Verification items for the finished model (mm, model axes). A direction names the side the tool comes from. Round coordinates to 2 decimals unless told otherwise and drop trailing zeros. Write each loop counter-clockwise with the first axis right and the second up, starting at its lowest first coordinate (ties: lowest second). Pieces come first, ordered by that corner, then holes. Notation, with made-up numbers: M -33.75,42.25 L -14.75,42.25 A14 ccw -14.75,52.25 Z; hole C 14,78 d7. An arc over 180 degrees is marked long. Answer in a Markdown table with one row per item. Add a question column.
1. Set-up check for faces 1 (the flat face through (-19, 1, 0)), 2 (the flat face through (-44, -8, 6.096)): record each of +Z, -Z, +X, -X, +Y, -Y from which the full face is reachable in a straight line by a thin tool's end or side.
2. Go/stop test with flat-tipped pins: pin 1 Ø2 at (x, z) = (-21.5, 1.5) entering from -Y; pin 2 Ø0.6 at (y, z) = (16, 6.5) entering from -X; pin 3 Ø0.6 at (y, z) = (30, 6.5) entering from -X. Record where each tip stops, or that it passes through.
3. Material ranges on probe 1 along Y at (x, z) = (-38, 6.25); probe 2 along Z at (x, y) = (13.5, -2); probe 3 along Z at (x, y) = (4, -14.5), recorded low to high.
4. Sectioned sample at A-A on y = 19. Record the cut outline in (x, z), plus the area to 3 significant figures.
5. Draft check along X on faces 3 (the flat face through (-55.315, 1.596, 3.219)), 4 (the flat face through (0, 21, 6.604)), 5 (the flat face through (-23, 13, 6.096)), 6 (the flat face through (-44, 28, 6.096)). Enter one of: pulls with the +X half, pulls with the -X half, needs draft (parallel to the pull), parting line crosses it, or undercut.
```python
from build123d import *

# Parameters (mm, degrees)
F0_W     = 38.1
F0_H     = 76.2
F1_DEPTH = 6.35
F3_DEPTH = 6.35
F5_W     = 8.6051712304
F5_H     = 10.1246496194
F6_DEPTH = 0.254
F8_DEPTH = 0.254


with BuildPart() as f1:
    # F0 (on Top) → F1 (new body)
    with BuildSketch(Plane.XY):
        Rectangle(F0_W, F0_H)
    extrude(amount=F1_DEPTH)

    # F2 (on face) → F3 (cut)
    with BuildSketch(Plane.XY.offset(6.35)):
        with BuildLine():
            Line((-3.9472845383, 38.1), (-3.8636967831, 38.1))
            add(Edge.make_bspline(
                [(-3.9472845383, 38.1), (-3.9204592136, 38.1251084892), (-3.8998782769, 38.127174182), (-3.8636967831, 38.1)],
                knots=[0.4563634252, 0.4563634252, 0.4563634252, 0.4563634252, 0.4871979804, 0.4871979804, 0.4871979804, 0.4871979804], degree=3))
        make_face()
        with BuildLine():
            add(Edge.make_bspline(
                [(-19.05, 32.5106605887), (-6.1091777888, 32.3092094071), (-4.3443097915, 37.7283845811), (-3.9472845383, 38.1)],
                knots=[0, 0, 0, 0, 0.4563634252, 0.4563634252, 0.4563634252, 0.4563634252], degree=3))
            Line((-3.9472845383, 38.1), (-19.05, 38.1))
            Line((-19.05, 38.1), (-19.05, 32.5106605887))
        make_face()
        with BuildLine():
            Line((19.05, -38.1), (19.05, 3.1485415529))
            Line((19.05, 3.1485415529), (15.3276119381, 0))
            add(Edge.make_bspline(
                [(15.3276119381, 0), (15.1655543596, -11.4850010723), (13.7070389464, -32.0684760809), (-13.3565291762, -32.3926247656)],
                knots=[0, 0, 0, 0, 43.2673328352, 43.2673328352, 43.2673328352, 43.2673328352], degree=3))
            Line((-13.3565291762, -32.3926247656), (-19.05, -38.1))
            Line((-19.05, -38.1), (19.05, -38.1))
        make_face()
        with BuildLine():
            Line((19.05, 3.1485415529), (19.05, 32.5106605887))
            ThreePointArc((19.05, 32.5106605887), (12.2820636744, 17.8296010708), (19.05, 3.1485415529))
        make_face()
        Polygon((15.2206547403, 38.1), (19.05, 32.5106605887), (19.05, 38.1), align=None)
        with BuildLine():
            add(Edge.make_bspline(
                [(-3.8636967831, 38.1), (-3.843737622, 38.0850096328), (-3.0988894532, 37.3648301618), (5.2937592339, 27.6119129043), (15.2206547403, 38.1)],
                knots=[0.4871979804, 0.4871979804, 0.4871979804, 0.4871979804, 0.5042075561, 1, 1, 1, 1], degree=3))
            Line((15.2206547403, 38.1), (-3.8636967831, 38.1))
        make_face()
    extrude(amount=-F3_DEPTH, mode=Mode.SUBTRACT)

    # F4: F1 across face


with BuildPart() as f1_1:
    add(f1.part)
    add(f1.part.mirror(Plane(origin=(-19.05, -2.7946697056, 3.175), x_dir=(0, -1, 0), z_dir=(-1, 0, 0))))

    # F5 (on face) → F6 (cut)
    with BuildSketch(Plane.XY.offset(6.35)):
        with BuildLine():
            ThreePointArc((-37.5772565603, 32.5917619335), (-45.671204203, 31.008244813), (-53.4049263852, 33.873389857))
            ThreePointArc((-53.4049263852, 33.873389857), (-50.1581802259, 29.7090041206), (-47.9535559256, 24.9107647687))
            Line((-47.9535559256, 24.9107647687), (-37.5772565603, 24.9107647687))
            Line((-37.5772565603, 24.9107647687), (-37.5772565603, 32.5917619335))
        make_face()
        with BuildLine():
            Line((-37.5772565603, 17.7330877632), (-46.8293691707, 17.7330877632))
            ThreePointArc((-46.8293691707, 17.7330877632), (-47.4515529833, 12.5316587806), (-49.2414900542, 7.6084381438))
            Line((-49.2414900542, 7.6084381438), (-37.5772565603, 7.6084381438))
            Line((-37.5772565603, 7.6084381438), (-37.5772565603, 17.7330877632))
        make_face()
        with Locations((-23.3525856152, 12.6707629535)):
            Rectangle(F5_W, F5_H)
        with BuildLine():
            add(Edge.make_bspline(
                [(-27.6551712304, 30.7719508767), (-25.0542603527, 29.9722405749), (-22.0663375313, 29.5693060648), (-19.05, 29.5798139295)],
                knots=[8.2498540023, 8.2498540023, 8.2498540023, 8.2498540023, 15.7954011192, 15.7954011192, 15.7954011192, 15.7954011192], degree=3))
            Line((-27.6551712304, 30.7719508767), (-27.6551712304, 24.9107647687))
            Line((-27.6551712304, 24.9107647687), (-19.05, 24.9107647687))
            Line((-19.05, 24.9107647687), (-19.05, 29.5798139295))
        make_face()
        with BuildLine():
            add(Edge.make_bspline(
                [(-14.7775728256, 29.8755089086), (-13.3218013512, 30.0752082684), (-11.9002315961, 30.3766424012), (-10.555408895, 30.7817886934)],
                knots=[19.3738855113, 19.3738855113, 19.3738855113, 19.3738855113, 23.0815953476, 23.0815953476, 23.0815953476, 23.0815953476], degree=3))
            Line((-14.7775728256, 29.8755089086), (-14.7775728256, 7.6084381438))
            Line((-14.7775728256, 7.6084381438), (-10.555408895, 7.6084381438))
            Line((-10.555408895, 7.6084381438), (-10.555408895, 30.7817886934))
        make_face()
        with BuildLine():
            add(Edge.make_bspline(
                [(-6.3332454301, 32.5660842134), (-5.2855915186, 33.1701122102), (-4.348215472, 33.8675739108), (-3.5563470113, 34.6601066929)],
                knots=[27.291897076, 27.291897076, 27.291897076, 27.291897076, 30.7735982336, 30.7735982336, 30.7735982336, 30.7735982336], degree=3))
            Line((-6.3332454301, 32.5660842134), (-6.3332454301, 7.6084381438))
            Line((-6.3332454301, 7.6084381438), (-2.1110819653, 7.6084381438))
            Line((-2.1110819653, 7.6084381438), (-2.1110819653, 33.5563536252))
            ThreePointArc((-2.1110819653, 33.5563536252), (-2.8501925125, 34.0866536733), (-3.5563470113, 34.6601066929))
        make_face()
        with BuildLine():
            ThreePointArc((6.3332458958, 30.9586713834), (4.2005089038, 31.1180342806), (2.1110812668, 31.5743847599))
            Line((2.1110812668, 31.5743847599), (2.1110812668, 7.6084381438))
            Line((2.1110812668, 7.6084381438), (6.3332458958, 7.6084381438))
            Line((6.3332458958, 7.6084381438), (6.3332458958, 30.9586713834))
        make_face()
        with BuildLine():
            Line((11.1414900542, 0), (2.5332975201, 0))
            Line((2.5332975201, 0), (2.5332975201, -21.0394149611))
            add(Edge.make_bspline(
                [(2.5332975201, -21.0394149611), (7.0844292813, -16.8218684935), (10.3040141885, -10.1988507211), (11.1414900542, 0)],
                knots=[0.7794890643, 0.7794890643, 0.7794890643, 0.7794890643, 1, 1, 1, 1], degree=3))
        make_face()
        with BuildLine():
            Line((-6.1221369542, 0), (-14.7775728256, 0))
            Line((-14.7775728256, 0), (-14.7775728256, -6.1859292111))
            ThreePointArc((-14.7775728256, -6.1859292111), (-12.0094062526, -9.1081265301), (-11.0027304346, -13.0053803252))
            ThreePointArc((-11.0027304346, -13.0053803252), (-12.0094062526, -16.9026341203), (-14.7775728256, -19.8248314393))
            Line((-14.7775728256, -19.8248314393), (-14.7775728256, -27.7072399522))
            add(Edge.make_bspline(
                [(-14.7775728256, -27.7072399522), (-11.7973621926, -27.4741929831), (-8.8730169385, -26.9647393053), (-6.1221369542, -26.0478686811)],
                knots=[0.5504848433, 0.5504848433, 0.5504848433, 0.5504848433, 0.6567583921, 0.6567583921, 0.6567583921, 0.6567583921], degree=3))
            Line((-6.1221369542, -26.0478686811), (-6.1221369542, 0))
        make_face()
        with BuildLine():
            Line((-23.4330072999, 0), (-32.0884436369, 0))
            Line((-32.0884436369, 0), (-32.0884436369, -26.0107606504))
            add(Edge.make_bspline(
                [(-32.0884436369, -26.0107606504), (-29.3393823668, -26.9395470029), (-26.4149145694, -27.4583082328), (-23.4330072999, -27.6984636108)],
                knots=[0.341816395, 0.341816395, 0.341816395, 0.341816395, 0.4482004295, 0.4482004295, 0.4482004295, 0.4482004295], degree=3))
            Line((-23.4330072999, -27.6984636108), (-23.4330072999, -19.7542909386))
            ThreePointArc((-23.4330072999, -19.7542909386), (-27.0972695654, -13.0053803252), (-23.4330072999, -6.2564697118))
            Line((-23.4330072999, -6.2564697118), (-23.4330072999, 0))
        make_face()
        with BuildLine():
            Line((-40.7438799739, 0), (-49.2414900542, 0))
            add(Edge.make_bspline(
                [(-49.2414900542, 0), (-48.410813311, -10.1160504409), (-45.236549248, -16.7140936827), (-40.7438799739, -20.9362171076)],
                knots=[0, 0, 0, 0, 0.218720698, 0.218720698, 0.218720698, 0.218720698], degree=3))
            Line((-40.7438799739, -20.9362171076), (-40.7438799739, 0))
        make_face()
    extrude(amount=-F6_DEPTH, mode=Mode.SUBTRACT)

    # F7 (on face) → F8 (join)
    with BuildSketch(Plane.XY.offset(6.35)):
        with BuildLine():
            Line((-40.7438799739, 0), (-40.7438799765, -20.9362171051))
            ThreePointArc((-40.7438799765, -20.9362171051), (-36.7357760167, -24.0186414564), (-32.0884436271, -26.0107606537))
            Line((-32.0884436271, -26.0107606537), (-32.0884436369, 0))
            Line((-32.0884436369, 0), (-40.7438799739, 0))
        make_face()
        with BuildLine():
            Line((-10.5554089048, 30.7817886905), (-10.555408895, 7.6084381438))
            Line((-10.555408895, 7.6084381438), (-6.3332454301, 7.6084381438))
            Line((-6.3332454301, 7.6084381438), (-6.3332454301, 32.5660842134))
            ThreePointArc((-6.3332454301, 32.5660842134), (-8.3220779988, 31.3846592732), (-10.5554089048, 30.7817886905))
        make_face()
        with BuildLine():
            Line((-2.1110819653, 33.5563536252), (-2.1110819653, 7.6084381438))
            Line((-2.1110819653, 7.6084381438), (2.1110812668, 7.6084381438))
            Line((2.1110812668, 7.6084381438), (2.1110812668, 31.5743847599))
            ThreePointArc((2.1110812668, 31.5743847599), (-0.1480933869, 32.2498884656), (-2.1110819653, 33.5563536252))
        make_face()
        Polygon((-19.05, 17.7330877632), (-19.05, 7.6084381438), (-14.7775728256, 7.6084381438), (-14.7775728256, 29.8755089086), (-19.05, 29.5798139295), (-19.05, 24.9107647687), align=None)
        with BuildLine():
            Line((-6.1221369542, 0), (-6.1221369542, -26.0478686811))
            ThreePointArc((-6.122136964, -26.0478686844), (-1.3860461596, -24.2493787213), (2.5332975225, -21.0394149589))
            Line((2.5332975201, -21.0394149611), (2.5332975201, 0))
            Line((2.5332975201, 0), (-6.1221369542, 0))
        make_face()
        with BuildLine():
            Line((-23.4330072999, -19.7542909386), (-23.4330072999, -27.6984636108))
            ThreePointArc((-23.4330072999, -27.6984636108), (-19.1056699461, -28.0775017142), (-14.7775728256, -27.7072399522))
            Line((-14.7775728256, -27.7072399522), (-14.7775728256, -19.8248314393))
            ThreePointArc((-14.7775728256, -19.8248314393), (-11.0027304346, -13.0053803252), (-14.7775728256, -6.1859292111))
            Line((-14.7775728256, -6.1859292111), (-14.7775728256, 0))
            Line((-14.7775728256, 0), (-23.4330072999, 0))
            Line((-23.4330072999, 0), (-23.4330072999, -6.2564697118))
            ThreePointArc((-23.4330072999, -6.2564697118), (-27.0972695654, -13.0053803252), (-23.4330072999, -19.7542909386))
        make_face()
        with BuildLine():
            Line((6.3332458958, 30.9586713834), (6.3332458958, 7.6084381438))
            Line((6.3332458958, 7.6084381438), (11.3998418674, 7.6084381438))
            ThreePointArc((11.3998418674, 7.6084381438), (9.3955290294, 20.8910955307), (13.7893487286, 33.5852125012))
            ThreePointArc((13.7893487286, 33.5852125012), (10.2858459166, 31.6345038021), (6.3332458958, 30.9586713834))
        make_face()
        with BuildLine():
            Line((-37.5772565603, 17.7330877632), (-37.5772565603, 7.6084381438))
            Line((-37.5772565603, 7.6084381438), (-27.6551712304, 7.6084381438))
            Line((-27.6551712304, 7.6084381438), (-27.6551712304, 17.7330877632))
            Line((-27.6551712304, 17.7330877632), (-19.05, 17.7330877632))
            Line((-19.05, 17.7330877632), (-19.05, 24.9107647687))
            Line((-19.05, 24.9107647687), (-27.6551712304, 24.9107647687))
            Line((-27.6551712304, 24.9107647687), (-27.6551712305, 30.7719508767))
            ThreePointArc((-27.6551712305, 30.7719508767), (-31.2495313727, 32.6633513709), (-34.2058315873, 35.4485101998))
            ThreePointArc((-34.2058315873, 35.4485101998), (-35.7322331398, 33.8321233993), (-37.5772565603, 32.5917619335))
            Line((-37.5772565603, 32.5917619335), (-37.5772565603, 24.9107647687))
            Line((-37.5772565603, 24.9107647687), (-47.9535559256, 24.9107647687))
            ThreePointArc((-47.9535559256, 24.9107647687), (-46.9346789734, 21.3934689174), (-46.8293691707, 17.7330877632))
            Line((-46.8293691707, 17.7330877632), (-37.5772565603, 17.7330877632))
        make_face()
    extrude(amount=F8_DEPTH)


solid = f1_1.part
```
Geometry check:
| question | item | result |
|---|---|---|
| 1 | face 1 | -Z, +X, -X, +Y, -Y |
| 1 | face 2 | +Z |
| 2 | pin 1 | stops at y = -36.65 |
| 2 | pin 2 | stops at x = -50.5 |
| 2 | pin 3 | stops at x = -54.92 |
| 3 | probe 1 | y = -30.04 to 7.61, 17.73 to 24.91, 32.39 to 34.93 |
| 3 | probe 2 | z = 0 to 6.35 |
| 3 | probe 3 | z = 0 to 6.1 |
| 4 | outline | M -50.42,0 L 12.32,0 L 12.32,6.35 L 9.29,6.35 L 9.29,6.6 L 6.33,6.6 L 6.33,6.1 L 2.11,6.1 L 2.11,6.6 L -2.11,6.6 L -2.11,6.1 L -6.33,6.1 L -6.33,6.6 L -10.56,6.6 L -10.56,6.1 L -14.78,6.1 L -14.78,6.6 L -46.76,6.6 L -46.76,6.35 L -50.42,6.35 Z |
| 4 | area | 406 mm2 |
| 5 | face 3 | pulls with the -X half |
| 5 | face 4 | needs draft |
| 5 | face 5 | undercut |
| 5 | face 6 | undercut |
